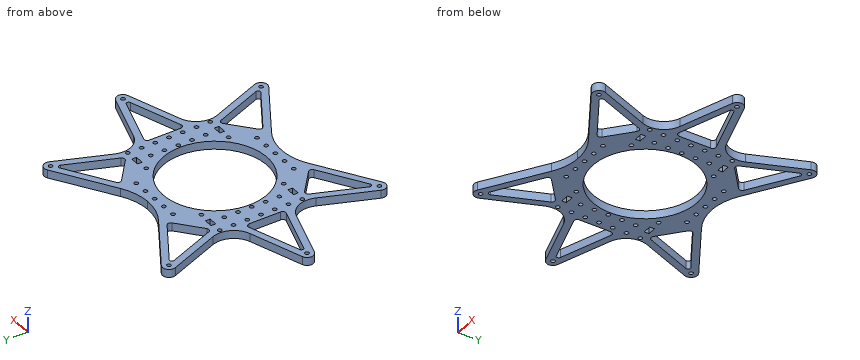
from build123d import *

# Parameters (mm, degrees)
SKETCH1_R           = 1.450000006
SKETCH1_R_2         = 1.45
SKETCH1_R_3         = 37.5
SKETCH1_W           = 6.2
SKETCH1_H           = 3.4
BOSS_EXTRUDE1_DEPTH = 5.85


with BuildPart() as part:
    # Sketch1 → Boss-Extrude1 (new body)
    with BuildSketch(Plane.XY):
        with BuildLine():
            Line((587.995290395, 497.753361998), (603.001149052, 460.347016836))
            ThreePointArc((603.001149052, 460.347016836), (602.663461243, 448.032016356), (593.446685098, 439.857402764))
            Line((593.446685098, 439.857402764), (555.146182231, 427.30822221))
            ThreePointArc((555.146182231, 427.30822221), (551.939243509, 422.882775531), (555.146182231, 418.457328853))
            Line((555.146182231, 418.457328853), (593.451704621, 405.906503648))
            ThreePointArc((593.451704621, 405.906503648), (602.672646523, 397.727172938), (603.008211739, 385.405865524))
            Line((603.008211739, 385.405865524), (587.996899243, 348.012788825))
            ThreePointArc((587.996899243, 348.012788825), (589.323611121, 342.712892318), (594.773109373, 342.32297413))
            Line((594.773109373, 342.32297413), (636.531879216, 368.248955529))
            ThreePointArc((636.531879216, 368.248955529), (646.164378733, 372.489187309), (656.596182238, 373.882775531))
            ThreePointArc((656.596182238, 373.882775531), (667.027985743, 372.489187309), (676.66048526, 368.248955529))
            Line((676.66048526, 368.248955529), (718.419255103, 342.32297413))
            ThreePointArc((718.419255103, 342.32297413), (723.868753355, 342.712892318), (725.195465233, 348.012788825))
            Line((725.195465233, 348.012788825), (710.184152737, 385.405865524))
            ThreePointArc((710.184152737, 385.405865524), (710.519717953, 397.727172938), (719.740659854, 405.906503648))
            Line((719.740659854, 405.906503648), (758.046182244, 418.457328853))
            ThreePointArc((758.046182244, 418.457328853), (761.253120966, 422.882775531), (758.046182244, 427.30822221))
            Line((758.046182244, 427.30822221), (719.745679378, 439.857402764))
            ThreePointArc((719.745679378, 439.857402764), (710.528903233, 448.032016356), (710.191215423, 460.347016836))
            Line((710.191215423, 460.347016836), (725.197074081, 497.753361998))
            ThreePointArc((725.197074081, 497.753361998), (723.86836572, 503.054641878), (718.416896408, 503.442606583))
            Line((718.416896408, 503.442606583), (677.369935548, 477.934266348))
            ThreePointArc((677.369935548, 477.934266348), (667.39800528, 473.484079569), (656.596182238, 471.882775531))
            ThreePointArc((656.596182238, 471.882775531), (645.794359196, 473.484079569), (635.822428927, 477.934266348))
            Line((635.822428927, 477.934266348), (594.775468067, 503.442606583))
            ThreePointArc((594.775468067, 503.442606583), (589.323998755, 503.054641878), (587.995290395, 497.753361998))
        make_face()
        with Locations((592.317421269, 499.487219843)):
            Circle(SKETCH1_R, mode=Mode.SUBTRACT)
        with Locations(Location((706.596182238, 432.882775531, 0), (0, 0, 180))):
            Circle(SKETCH1_R_2, mode=Mode.SUBTRACT)
        with Locations(Location((706.596182238, 442.882775531, 0), (0, 0, 180))):
            Circle(SKETCH1_R_2, mode=Mode.SUBTRACT)
        with Locations(Location((706.596182238, 452.882775531, 0), (0, 0, 180))):
            Circle(SKETCH1_R_2, mode=Mode.SUBTRACT)
        with Locations((706.596182238, 392.882775531)):
            Circle(SKETCH1_R_2, mode=Mode.SUBTRACT)
        with Locations((556.596182238, 422.882775531)):
            Circle(SKETCH1_R, mode=Mode.SUBTRACT)
        with Locations(Location((646.596182238, 378.882775531, 0), (0, 0, 180))):
            Circle(SKETCH1_R_2, mode=Mode.SUBTRACT)
        with Locations((656.596182238, 422.882775531)):
            Circle(SKETCH1_R_3, mode=Mode.SUBTRACT)
        with Locations(Location((636.596182238, 378.882775531, 0), (0, 0, 180))):
            Circle(SKETCH1_R_2, mode=Mode.SUBTRACT)
        with Locations((706.596182238, 402.882775531)):
            Circle(SKETCH1_R_2, mode=Mode.SUBTRACT)
        with Locations((656.596182238, 466.882775531)):
            Circle(SKETCH1_R_2, mode=Mode.SUBTRACT)
        with Locations(Location((696.596182238, 432.882775531, 0), (0, 0, 180))):
            Circle(SKETCH1_R_2, mode=Mode.SUBTRACT)
        with Locations((592.317421269, 346.278331219)):
            Circle(SKETCH1_R, mode=Mode.SUBTRACT)
        with Locations((706.596182238, 412.882775531)):
            Circle(SKETCH1_R_2, mode=Mode.SUBTRACT)
        with Locations(Location((656.596182238, 378.882775531, 0), (0, 0, 180))):
            Circle(SKETCH1_R_2, mode=Mode.SUBTRACT)
        with Locations(Location((696.596182238, 442.882775531, 0), (0, 0, 180))):
            Circle(SKETCH1_R_2, mode=Mode.SUBTRACT)
        with Locations((696.596182238, 402.882775531)):
            Circle(SKETCH1_R_2, mode=Mode.SUBTRACT)
        with Locations((696.596182238, 412.882775531)):
            Circle(SKETCH1_R_2, mode=Mode.SUBTRACT)
        with Locations((646.596182238, 466.882775531)):
            Circle(SKETCH1_R_2, mode=Mode.SUBTRACT)
        with Locations((636.596182238, 466.882775531)):
            Circle(SKETCH1_R_2, mode=Mode.SUBTRACT)
        with Locations(Location((696.596182238, 422.882775531, 0), (0, 0, 180))):
            Circle(SKETCH1_R_2, mode=Mode.SUBTRACT)
        with Locations(Location((676.596182238, 466.882775531, 0), (0, 0, 180))):
            Circle(SKETCH1_R_2, mode=Mode.SUBTRACT)
        with Locations(Location((666.596182238, 466.882775531, 0), (0, 0, 180))):
            Circle(SKETCH1_R_2, mode=Mode.SUBTRACT)
        with Locations(Location((706.596182238, 422.882775531, 0), (0, 0, 180))):
            Circle(SKETCH1_R_2, mode=Mode.SUBTRACT)
        with Locations(Location((686.596182238, 452.882775531, 0), (0, 0, 180))):
            Circle(SKETCH1_R_2, mode=Mode.SUBTRACT)
        with Locations((686.596182238, 392.882775531)):
            Circle(SKETCH1_R_2, mode=Mode.SUBTRACT)
        with Locations(Location((626.596182238, 392.882775531, 0), (0, 0, 180))):
            Circle(SKETCH1_R_2, mode=Mode.SUBTRACT)
        with Locations(Location((720.874943207, 346.278331219, 0), (0, 0, 180))):
            Circle(SKETCH1_R, mode=Mode.SUBTRACT)
        with Locations((676.596182238, 378.882775531)):
            Circle(SKETCH1_R_2, mode=Mode.SUBTRACT)
        with Locations((666.596182238, 378.882775531)):
            Circle(SKETCH1_R_2, mode=Mode.SUBTRACT)
        with Locations(Location((756.596182238, 422.882775531, 0), (0, 0, 180))):
            Circle(SKETCH1_R, mode=Mode.SUBTRACT)
        with Locations((626.596182238, 452.882775531)):
            Circle(SKETCH1_R_2, mode=Mode.SUBTRACT)
        with Locations((606.596182238, 422.882775531)):
            Circle(SKETCH1_R_2, mode=Mode.SUBTRACT)
        with Locations((616.596182238, 422.882775531)):
            Circle(SKETCH1_R_2, mode=Mode.SUBTRACT)
        with Locations(Location((616.596182238, 412.882775531, 0), (0, 0, 180))):
            Circle(SKETCH1_R_2, mode=Mode.SUBTRACT)
        with Locations(Location((720.874943207, 499.487219843, 0), (0, 0, 180))):
            Circle(SKETCH1_R, mode=Mode.SUBTRACT)
        with Locations(Location((616.596182238, 402.882775531, 0), (0, 0, 180))):
            Circle(SKETCH1_R_2, mode=Mode.SUBTRACT)
        with Locations((616.596182238, 442.882775531)):
            Circle(SKETCH1_R_2, mode=Mode.SUBTRACT)
        with Locations(Location((606.596182238, 412.882775531, 0), (0, 0, 180))):
            Circle(SKETCH1_R_2, mode=Mode.SUBTRACT)
        with Locations((616.596182238, 432.882775531)):
            Circle(SKETCH1_R_2, mode=Mode.SUBTRACT)
        with Locations(Location((606.596182238, 402.882775531, 0), (0, 0, 180))):
            Circle(SKETCH1_R_2, mode=Mode.SUBTRACT)
        with Locations(Location((606.596182238, 392.882775531, 0), (0, 0, 180))):
            Circle(SKETCH1_R_2, mode=Mode.SUBTRACT)
        with Locations((606.596182238, 452.882775531)):
            Circle(SKETCH1_R_2, mode=Mode.SUBTRACT)
        with Locations((606.596182238, 442.882775531)):
            Circle(SKETCH1_R_2, mode=Mode.SUBTRACT)
        with Locations((606.596182238, 432.882775531)):
            Circle(SKETCH1_R_2, mode=Mode.SUBTRACT)
        with BuildLine():
            Line((594.852213644, 494.089955534), (608.761050105, 459.418248349))
            ThreePointArc((608.761050105, 459.418248349), (610.328090614, 458.05093997), (612.354775393, 458.517520045))
            Line((612.354775393, 458.517520045), (629.185249241, 472.639964443))
            ThreePointArc((629.185249241, 472.639964443), (629.996671034, 474.554838547), (628.922248871, 476.335502797))
            Line((628.922248871, 476.335502797), (597.192526929, 496.053711548))
            ThreePointArc((597.192526929, 496.053711548), (595.310843783, 495.919797808), (594.852213644, 494.089955534))
        make_face(mode=Mode.SUBTRACT)
        with Locations((696.596182238, 392.882775531)):
            Rectangle(SKETCH1_W, SKETCH1_H, mode=Mode.SUBTRACT)
        with BuildLine():
            Line((562.360059701, 421.35524452), (599.360059701, 409.232174436))
            ThreePointArc((599.360059701, 409.232174436), (601.41475291, 409.553708225), (602.360059701, 411.406150729))
            Line((602.360059701, 411.406150729), (602.360059701, 434.359400333))
            ThreePointArc((602.360059701, 434.359400333), (601.41475291, 436.211842837), (599.360059701, 436.533376627))
            Line((599.360059701, 436.533376627), (562.360059701, 424.410306542))
            ThreePointArc((562.360059701, 424.410306542), (561.253120966, 422.882775531), (562.360059701, 421.35524452))
        make_face(mode=Mode.SUBTRACT)
        with BuildLine():
            Line((594.897239667, 351.78038038), (608.794032765, 386.397196889))
            ThreePointArc((608.794032765, 386.397196889), (610.36130643, 387.761102695), (612.3843749, 387.288049044))
            Line((612.3843749, 387.288049044), (629.156141394, 373.086154531))
            ThreePointArc((629.156141394, 373.086154531), (629.961681006, 371.166639364), (628.883661612, 369.385823055))
            Line((628.883661612, 369.385823055), (597.19261369, 349.710398658))
            ThreePointArc((597.19261369, 349.710398658), (595.266724956, 349.882452422), (594.897239667, 351.78038038))
        make_face(mode=Mode.SUBTRACT)
        with Locations((616.596182238, 452.882775531)):
            Rectangle(SKETCH1_W, SKETCH1_H, mode=Mode.SUBTRACT)
        with Locations((696.596182238, 452.882775531)):
            Rectangle(SKETCH1_W, SKETCH1_H, mode=Mode.SUBTRACT)
        with BuildLine():
            Line((715.999750786, 349.710398658), (684.308702864, 369.385823055))
            ThreePointArc((684.308702864, 369.385823055), (683.230683469, 371.166639364), (684.036223082, 373.086154531))
            Line((684.036223082, 373.086154531), (700.807989576, 387.288049044))
            ThreePointArc((700.807989576, 387.288049044), (702.831058046, 387.761102695), (704.39833171, 386.397196889))
            Line((704.39833171, 386.397196889), (718.295124809, 351.78038038))
            ThreePointArc((718.295124809, 351.78038038), (717.92563952, 349.882452422), (715.999750786, 349.710398658))
        make_face(mode=Mode.SUBTRACT)
        with BuildLine():
            Line((750.832304774, 424.410306542), (713.832304774, 436.533376627))
            ThreePointArc((713.832304774, 436.533376627), (711.777611566, 436.211842837), (710.832304774, 434.359400333))
            Line((710.832304774, 434.359400333), (710.832304774, 411.406150729))
            ThreePointArc((710.832304774, 411.406150729), (711.777611565, 409.553708225), (713.832304774, 409.232174436))
            Line((713.832304774, 409.232174436), (750.832304774, 421.35524452))
            ThreePointArc((750.832304774, 421.35524452), (751.939243509, 422.882775531), (750.832304774, 424.410306542))
        make_face(mode=Mode.SUBTRACT)
        with BuildLine():
            Line((684.007115235, 472.639964443), (700.837589083, 458.517520045))
            ThreePointArc((700.837589083, 458.517520045), (702.864273862, 458.05093997), (704.431314371, 459.418248349))
            Line((704.431314371, 459.418248349), (718.340150832, 494.089955534))
            ThreePointArc((718.340150832, 494.089955534), (717.881520693, 495.919797808), (715.999837547, 496.053711548))
            Line((715.999837547, 496.053711548), (684.270115605, 476.335502797))
            ThreePointArc((684.270115605, 476.335502797), (683.195693441, 474.554838547), (684.007115235, 472.639964443))
        make_face(mode=Mode.SUBTRACT)
        with Locations((616.596182238, 392.882775531)):
            Rectangle(SKETCH1_W, SKETCH1_H, mode=Mode.SUBTRACT)
    extrude(amount=BOSS_EXTRUDE1_DEPTH)


solid = part.part
The listing builds one solid part. Answer for the finished solid, in the listing's coordinates (mm). Coordinates: 2 decimals unless noted, no trailing zeros. Write each loop counter-clockwise with the first axis right and the second up, starting at its lowest first coordinate (ties: lowest second). Pieces come first, ordered by that corner, then holes. Notation, with made-up numbers: (64.25, 62.5) - (111.25, 62.5) arc R8 cw to (111.25, 69.5) - close; hole circle Ø1 at (8.25, 14.5). An arc over 180 degrees is marked (long way). Answer as CSV lines item,"result".
1. Find section C-C (z = 4.4). Give the number of separate pieces and of enclosed holes in the cut face, plus the area to 3 significant figures.
Computed values:
separate pieces,"1"
enclosed holes,"55"
area,"8,120 mm²"
2. Given P1, Ø3.5, axis at y = 393, z = 2.5, coming from the -X side; P2, Ø1.8, axis at x = 616, z = 3.5, coming from the +Y side; P3, Ø3.5, axis at y = 453.5, z = 2, coming from the +X side, each flat-ended and moving along its own axis, determine where each tip first touches the part or whether it passes through.
Computed values:
P1,"stops at x = 603.71"
P2,"stops at y = 490.81"
P3,"stops at x = 709.34"
3. Straight lines are drawn through the part: line 1 (Y direction, x = 713, z = 3.4); line 2 (X direction, y = 493, z = 5.35); line 3 (X direction, y = 383, z = 1.2). For each, find the intervals that lie inside material, in ascending order. Write a range as [from, to].
Computed values:
line 1,"y = [345.69, 351.57], [364.97, 378.39], [401.49, 409.12], [436.64, 444.28], [467.35, 480.78], [494.19, 500.08]"
line 2,"x = [589.9, 595.29], [602.11, 611.58], [701.61, 711.09], [717.9, 723.29]"
line 3,"x = [602.04, 607.43], [617.45, 695.74], [705.76, 711.15]"
4. Find section B-B (y = 449). Give the vertices of the cut face in (x, z), plus the area to 3 significant figures.
Computed values:
outline,"(603.08, 0) - (629.69, 0) - (629.69, 5.85) - (603.08, 5.85) - close; (683.51, 0) - (710.12, 0) - (710.12, 5.85) - (683.51, 5.85) - close"
area,"311 mm²"
5. Find section D-D (y = 485). Give the vertices of the cut face in (x, z), plus the area to 3 significant figures.
Computed values:
outline,"(593.11, 0) - (598.5, 0) - (598.5, 5.85) - (593.11, 5.85) - close; (614.98, 0) - (624.45, 0) - (624.45, 5.85) - (614.98, 5.85) - close; (688.74, 0) - (698.21, 0) - (698.21, 5.85) - (688.74, 5.85) - close; (714.69, 0) - (720.08, 0) - (720.08, 5.85) - (714.69, 5.85) - close"
area,"174 mm²"
6. Find section A-A (y = 363.5). Give the vertices of the cut face in (x, z), plus the area to 3 significant figures.
Computed values:
outline,"(594.21, 0) - (599.6, 0) - (599.6, 5.85) - (594.21, 5.85) - close; (619.4, 0) - (628.88, 0) - (628.88, 5.85) - (619.4, 5.85) - close; (684.31, 0) - (693.79, 0) - (693.79, 5.85) - (684.31, 5.85) - close; (713.59, 0) - (718.98, 0) - (718.98, 5.85) - (713.59, 5.85) - close"
area,"174 mm²"
